from build123d import *

# Parameters (mm, degrees)
BOSS_EXTRUDE2_DEPTH                = 38.1
F_5_16_0_3125_DIAMETER_HOLE1_D     = 7.9375
F_5_16_0_3125_DIAMETER_HOLE1_DEPTH = 3.175


with BuildPart() as part:
    # Sketch1 → Boss-Extrude2 (new body, symmetric)
    with BuildSketch(Plane(origin=(0, 0, 0), x_dir=(0, 0, -1), z_dir=(1, 0, 0))):
        Polygon((0, 0), (-25.4, 0), (-25.4, -3.175), (-3.175, -3.175), (-3.175, -25.4), (0, -25.4), align=None)
    extrude(amount=BOSS_EXTRUDE2_DEPTH, both=True)

    # 5/16 (0.3125) Diameter Hole1
    with Locations(Plane(origin=(0, 0, 0), x_dir=(1, 0, 0), z_dir=(0, 1, 0))):
        with Locations((-26.9875, -14.2875), (26.9875, -14.2875)):
            Hole(F_5_16_0_3125_DIAMETER_HOLE1_D / 2, depth=F_5_16_0_3125_DIAMETER_HOLE1_DEPTH)


solid = part.part
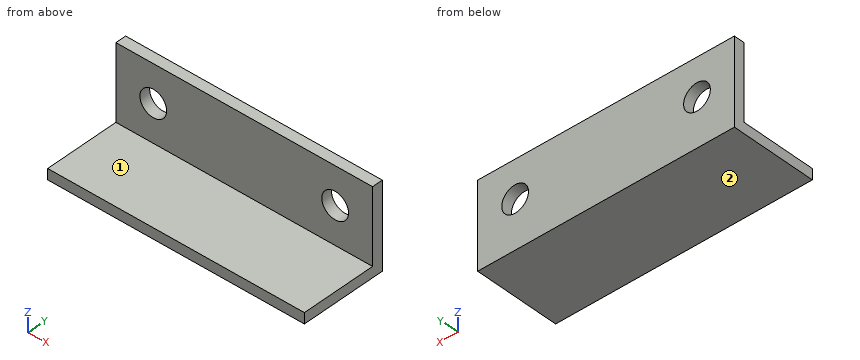
The model under review builds one solid part; all positions refer to its coordinate system, in mm. Face numbers are marked on the shaded views. A direction names the side the tool comes from. Give positions to 0.01 mm unless a question says otherwise; leave off trailing zeros. Order: outer loops, then holes, each group sorted by start corner. A loop starts at its lowest first (then second) coordinate and runs counter-clockwise, first axis right, second up. Notation, with made-up numbers: M 33,84 L 80,84 A23 cw 80,107 Z; hole C -36,-17 d4. An arc over 180 degrees is marked long. Answer in a Markdown table with one row per item. Add a question column.
1. Add section C-C on y = -17. State the section outline as (x, z) points (3 decimals), plus the area to 3 significant figures.
2. To check wall thickness, follow line 1 along Y through (x, z) = (-8, 11.5) (3 decimals); line 2 along Z through (x, y) = (34, -13.25) (3 decimals). State the ranges of each line that lie inside material, in increasing order.
3. For pin 1 Ø1 at (x, z) = (6.5, 12.5) entering from -Y (3 decimals); pin 2 Ø2 at (x, z) = (-29.5, 14) entering from +Y, all flat-tipped, find the tip position at first contact; note any pin that passes through.
4. Machinability: for the marked faces 1 and 2, which of the approach directions +Z, -Z, +X, -X, +Y, -Y give a long, thin tool a straight path to every point of the face, cutting with its end or side? Answer none if there is none.
5. Add section A-A on x = -11. State the section outline as (y, z) points (3 decimals).
6. Add section B-B on z = 20.5. State the section outline as (x, y) points (3 decimals), plus the area to 3 significant figures.
The answers:
| question | item | result |
|---|---|---|
| 1 | outline | M -38.1,0 L 38.1,0 L 38.1,3.175 L -38.1,3.175 Z |
| 1 | area | 242 mm2 |
| 2 | line 1 | -3.175 to 0 |
| 2 | line 2 | 0 to 3.175 |
| 3 | pin 1 | y = -3.175 |
| 3 | pin 2 | through |
| 4 | face 1 | +Z, +X, -X, -Y |
| 4 | face 2 | -Z, +X, -X, +Y, -Y |
| 5 | outline | M -25.4,0 L 0,0 L 0,25.4 L -3.175,25.4 L -3.175,3.175 L -25.4,3.175 Z |
| 6 | outline | M -38.1,-3.175 L 38.1,-3.175 L 38.1,0 L -38.1,0 Z |
| 6 | area | 242 mm2 |
